Part model, mm, in its own coordinate system. A direction names the side the tool comes from. Round coordinates to 2 decimals unless told otherwise and drop trailing zeros. Write each loop counter-clockwise with the first axis right and the second up, starting at its lowest first coordinate (ties: lowest second). Pieces come first, ordered by that corner, then holes.
```python
from build123d import *

# Parameters (mm, degrees)
BOSS_EXTRUDE1_DEPTH = 3
SKETCH2_W           = 0.5
SKETCH2_H           = 0.5
BOSS_EXTRUDE2_DEPTH = 10
CHAMFER1_SIZE       = 0.1


with BuildPart() as part:
    # Sketch1 → Boss-Extrude1 (new body)
    with BuildSketch(Plane(origin=(0, 0, 0), x_dir=(1, 0, 0), z_dir=(0, 1, 0))):
        Polygon((-5, 44.5), (-25.5, 35.5), (25.5, 35.5), (5, 44.5), align=None)
        Polygon((-25.5, 35.5), (-35.5, 35.5), (-35.5, -35.5), (35.5, -35.5), (35.5, 35.5), (25.5, 35.5), align=None)
    extrude(amount=BOSS_EXTRUDE1_DEPTH)

    # Sketch2 → Boss-Extrude2 (add)
    with BuildSketch(Plane(origin=(0, 0, -44.5), x_dir=(-1, 0, 0), z_dir=(0, 0, -1))):
        with Locations((-3.81, 1.5)):
            Rectangle(SKETCH2_W, SKETCH2_H)
        with Locations((-1.27, 1.5)):
            Rectangle(SKETCH2_W, SKETCH2_H)
        with Locations((1.27, 1.5)):
            Rectangle(SKETCH2_W, SKETCH2_H)
        with Locations((3.81, 1.5)):
            Rectangle(SKETCH2_W, SKETCH2_H)
    extrude(amount=BOSS_EXTRUDE2_DEPTH)

    # Chamfer1
    chamfer1_edges = [part.edges().sort_by_distance(p)[0] for p in [
        (3.56, 1.5, -44.5),
        (3.56, 1.25, -49.5),
        (3.81, 1.75, -44.5),
        (3.56, 1.75, -49.5),
        (4.06, 1.5, -44.5),
        (4.06, 1.75, -49.5),
        (3.81, 1.25, -44.5),
        (4.06, 1.25, -49.5),
        (3.56, 1.5, -54.5),
        (3.81, 1.75, -54.5),
        (4.06, 1.5, -54.5),
        (3.81, 1.25, -54.5),
        (1.02, 1.5, -44.5),
        (1.02, 1.25, -49.5),
        (1.27, 1.75, -44.5),
        (1.02, 1.75, -49.5),
        (1.52, 1.5, -44.5),
        (1.52, 1.75, -49.5),
        (1.27, 1.25, -44.5),
        (1.52, 1.25, -49.5),
        (1.02, 1.5, -54.5),
        (1.27, 1.75, -54.5),
        (1.52, 1.5, -54.5),
        (1.27, 1.25, -54.5),
        (-1.52, 1.5, -44.5),
        (-1.52, 1.25, -49.5),
        (-1.27, 1.75, -44.5),
        (-1.52, 1.75, -49.5),
        (-1.02, 1.5, -44.5),
        (-1.02, 1.75, -49.5),
        (-1.27, 1.25, -44.5),
        (-1.02, 1.25, -49.5),
        (-1.52, 1.5, -54.5),
        (-1.27, 1.75, -54.5),
        (-1.02, 1.5, -54.5),
        (-1.27, 1.25, -54.5),
        (-4.06, 1.5, -44.5),
        (-4.06, 1.25, -49.5),
        (-3.81, 1.75, -44.5),
        (-4.06, 1.75, -49.5),
        (-3.56, 1.5, -44.5),
        (-3.56, 1.75, -49.5),
        (-3.81, 1.25, -44.5),
        (-3.56, 1.25, -49.5),
        (-4.06, 1.5, -54.5),
        (-3.81, 1.75, -54.5),
        (-3.56, 1.5, -54.5),
        (-3.81, 1.25, -54.5),
    ]]
    chamfer(chamfer1_edges, length=CHAMFER1_SIZE)


solid = part.part
```
Q1. Which spindle directions (+Z, -Z, +X, -X, +Y, -Y) get a long thin tool onto all of the face, cutting with end or side? Do faces 1 (the flat face through (31, 1, -35.5)), 2 (the flat face through (0, 0, -5)). Say none if no direction does.
Values follow:
face 1: -Z, +X, +Y, -Y
face 2: +Z, -Z, +X, -X, -Y
Q2. Mould opens along X. For faces 3 (the flat face through (0, 1, -44.5)), 4 (the flat face through (-30, 1, -35.5)), 5 (the flat face through (-35.5, 1, 0)) say: +X half, -X half, draft (parallel to the pull), parting line (faces both ways), or undercut.
Values follow:
face 3: undercut
face 4: draft
face 5: -X half
Q3. Cut at B-B on z = -37.5. Write the cut outline in (x, y).
Values follow:
outline: (-20.94, 0) - (20.94, 0) - (20.94, 3) - (-20.94, 3) - close
Q4. Wall check: L1, parallel to Z at x = -0.5, y = 2.7; L2, parallel to Z at x = 30, y = 2.2; L3, parallel to X at y = 1.6, z = -43. Give the ranges that are in metal, low to high.
Values follow:
L1: z = -44.5 to 35.5
L2: z = -35.5 to 35.5
L3: x = -8.42 to 8.42
Q5. Drop a flat-ended pin along its axis: pin 1 (0.9 mm diameter, centred on x = -32, y = 2, fed in from -Z). Give the stop position or say it passes through.
Values follow:
pin 1: stops at z = -35.5
Q6. Cut at A-A on x = -6. Write the cut outline in (y, z).
Values follow:
outline: (0, -44.06) - (3, -44.06) - (3, 35.5) - (0, 35.5) - close
